from build123d import *

# Parameters (mm, degrees)
SKETCH1_W                  = 99
SKETCH1_H                  = 99
BOSS_EXTRUDE1_DEPTH        = 0.5
CUT_EXTRUDE1_DEPTH         = 71.010713466
M1_6_CLEARANCE_HOLE1_D     = 1.8
M1_6_CLEARANCE_HOLE1_DEPTH = 3
M1_6_CLEARANCE_HOLE1_TIP   = 0.540774557
FILLET1_R                  = 0.5


with BuildPart() as part:
    # Sketch1 → Boss-Extrude1 (new, symmetric)
    with BuildSketch(Plane.XY):
        Rectangle(SKETCH1_W, SKETCH1_H)
    extrude(amount=BOSS_EXTRUDE1_DEPTH, both=True)

    # Sketch2 → Cut-Extrude1 (cut, through all)
    with BuildSketch(Plane.XY.offset(0.5)):
        with BuildLine():
            Line((-49.5, 49.5), (-41, 49.5))
            Line((-41, 49.5), (-41, 42.5))
            ThreePointArc((-41, 42.5), (-41.439339828, 41.439339828), (-42.5, 41))
            Line((-42.5, 41), (-49.5, 41))
            Line((-49.5, 41), (-49.5, 49.5))
        make_face()
        with BuildLine():
            Line((49.5, 49.5), (41, 49.5))
            Line((41, 49.5), (41, 42.5))
            ThreePointArc((41, 42.5), (41.439339828, 41.439339828), (42.5, 41))
            Line((42.5, 41), (49.5, 41))
            Line((49.5, 41), (49.5, 49.5))
        make_face()
        with BuildLine():
            Line((-49.5, -49.5), (-41, -49.5))
            Line((-41, -49.5), (-41, -42.5))
            ThreePointArc((-41, -42.5), (-41.439339828, -41.439339828), (-42.5, -41))
            Line((-42.5, -41), (-49.5, -41))
            Line((-49.5, -41), (-49.5, -49.5))
        make_face()
        with BuildLine():
            Line((49.5, -49.5), (41, -49.5))
            Line((41, -49.5), (41, -42.5))
            ThreePointArc((41, -42.5), (41.439339828, -41.439339828), (42.5, -41))
            Line((42.5, -41), (49.5, -41))
            Line((49.5, -41), (49.5, -49.5))
        make_face()
    extrude(amount=-CUT_EXTRUDE1_DEPTH, mode=Mode.SUBTRACT)

    # M1.6 Clearance Hole1
    with Locations(Plane.XY.offset(0.5)):
        with Locations((-45.75, 29), (-29, 45.75), (29, 45.75), (45.75, 29), (45.75, -29), (29, -45.75), (-29, -45.75), (-45.75, -29)):
            Hole(M1_6_CLEARANCE_HOLE1_D / 2, depth=M1_6_CLEARANCE_HOLE1_DEPTH)
            with Locations((0, 0, -(M1_6_CLEARANCE_HOLE1_DEPTH + M1_6_CLEARANCE_HOLE1_TIP / 2))):  # 118° drill point
                Cone(0, M1_6_CLEARANCE_HOLE1_D / 2, M1_6_CLEARANCE_HOLE1_TIP, mode=Mode.SUBTRACT)

    # Fillet1
    fillet1_edges = [part.edges().sort_by_distance(p)[0] for p in [
        (-49.5, 0, 0.5),
        (-46, 41, 0.5),
        (-41.439339828, 41.439339828, 0.5),
        (-41, 46, 0.5),
        (0, 49.5, 0.5),
        (41.439339828, 41.439339828, 0.5),
        (46, 41, 0.5),
        (41, 46, 0.5),
        (49.5, 0, 0.5),
        (41.439339828, -41.439339828, 0.5),
        (41, -46, 0.5),
        (46, -41, 0.5),
        (0, -49.5, 0.5),
        (-41, -46, 0.5),
        (-41.439339828, -41.439339828, 0.5),
        (-46, -41, 0.5),
    ]]
    fillet(fillet1_edges, radius=FILLET1_R)


solid = part.part
Can you work these out from the model? Positions are in its coordinate system, mm. Coordinates: 2 decimals unless noted, no trailing zeros. Write each question's results on one line, items separated by ' | '. Start each with the question number.
Item 1: I'm going to push a flat-ended pin straight in: P1, Ø0.6, axis at x = -45, z = -0.5, coming from the +Y side. Where does the tip first touch, or does it pass through?
Item 2: If we section it at A-A, the plane z = -0.25: Count the separate pieces of the cut face and the enclosed holes in it, and give its area (3 significant figures).
Item 3: Please list where these lines run through material, in increasing order: probe 1 along Y at (x, z) = (29, -0.1); probe 2 along X at (y, z) = (-45.75, -0.2).
Answer block:
1) P1: y = 41
2) separate pieces: 1 | enclosed holes: 8 | area: 9,490 mm²
3) probe 1: -49.5 to -46.65, -44.85 to 44.85, 46.65 to 49.5 | probe 2: -41 to -29.9, -28.1 to 28.1, 29.9 to 41
